from build123d import *

# Parameters (mm, degrees)
F1_DEPTH = 6.35
F2_R     = 0.762
F4_DEPTH = 6.3510001


with BuildPart() as f1:
    # F0 (on Top) → F1 (new body)
    with BuildSketch(Plane.XY):
        with BuildLine():
            Line((4.7625, 16.3680184094), (-4.7625, 16.3680184094))
            Line((-4.7625, 16.3680184094), (-4.7625, 11.2880184094))
            Line((-4.7625, 11.2880184094), (-1.27, 11.2880184094))
            Line((-1.27, 11.2880184094), (-1.27, 4.9380184094))
            ThreePointArc((-1.27, 4.9380184094), (-6.4291435291, 3.7546941592), (-10.16, 0))
            add(Edge.make_bspline(
                [(-8.7527767482, 0), (-8.8089559621, -0.2418498758), (-9.0471031461, -0.7278683078), (-10.0843877691, -0.5834050266), (-10.1370594903, -0.1969189085), (-10.16, 0)],
                knots=[0, 0, 0, 0, 0.3394019143, 0.707080255, 1, 1, 1, 1], degree=3))
            ThreePointArc((-8.7527767482, 0), (-5.3825469605, 2.5206872974), (-1.27, 3.4147067439))
            Line((-1.27, 3.4147067439), (-1.27, -12.192))
            Line((-1.27, -12.192), (-1.778, -12.192))
            Line((-1.778, -12.192), (-6.223, -3.556))
            Line((-6.223, -3.556), (-6.223, -1.27))
            Line((-6.223, -1.27), (-6.985, -1.27))
            Line((-6.985, -1.27), (-6.985, -3.556))
            Line((-6.985, -3.556), (-8.001, -3.556))
            Line((-8.001, -3.556), (-2.54, -13.716))
            Line((-2.54, -13.716), (2.54, -13.716))
            Line((2.54, -13.716), (8.001, -3.556))
            Line((8.001, -3.556), (6.985, -3.556))
            Line((6.985, -3.556), (6.985, -1.27))
            Line((6.985, -1.27), (6.223, -1.27))
            Line((6.223, -1.27), (6.223, -3.556))
            Line((6.223, -3.556), (1.778, -12.192))
            Line((1.778, -12.192), (1.27, -12.192))
            Line((1.27, -12.192), (1.27, 3.4147067439))
            ThreePointArc((1.27, 3.4147067439), (5.3825469605, 2.5206872974), (8.7527767482, 0))
            add(Edge.make_bspline(
                [(8.7527767482, 0), (8.8795025593, -0.2082938871), (9.0832410123, -0.668988318), (10.0510359017, -0.7151657897), (10.232657896, -0.2924908845), (10.16, 0)],
                knots=[0, 0, 0, 0, 0.3352638068, 0.68469439, 1, 1, 1, 1], degree=3))
            ThreePointArc((10.16, 0), (6.4291435291, 3.7546941592), (1.27, 4.9380184094))
            Line((1.27, 4.9380184094), (1.27, 11.2880184094))
            Line((1.27, 11.2880184094), (4.7625, 11.2880184094))
            Line((4.7625, 11.2880184094), (4.7625, 16.3680184094))
        make_face()
    extrude(amount=F1_DEPTH)

    # F2
    f2_edges = [f1.edges().sort_by_distance(p)[0] for p in [
        (-2.54, -13.716, 3.175),
        (2.54, -13.716, 3.175),
        (-4.7625, 16.368018, 3.175),
        (-4.7625, 11.288018, 3.175),
        (4.7625, 16.368018, 3.175),
        (4.7625, 11.288018, 3.175),
        (1.27, 3.414707, 3.175),
        (8.752777, 0, 3.175),
        (-8.752777, 0, 3.175),
        (-1.27, 3.414707, 3.175),
    ]]
    fillet(f2_edges, radius=F2_R)

    # F3 (on face) → F4 (cut, through all)
    with BuildSketch(Plane.XY.offset(6.35)):
        with BuildLine():
            Line((-3.048, 12.2405184094), (3.048, 12.2405184094))
            ThreePointArc((3.048, 12.2405184094), (3.5868153673, 12.4637030421), (3.81, 13.0025184094))
            Line((3.81, 13.0025184094), (3.81, 14.6535184094))
            ThreePointArc((3.81, 14.6535184094), (3.5868153673, 15.1923337767), (3.048, 15.4155184094))
            Line((3.048, 15.4155184094), (-3.048, 15.4155184094))
            ThreePointArc((-3.048, 15.4155184094), (-3.5868153673, 15.1923337767), (-3.81, 14.6535184094))
            Line((-3.81, 14.6535184094), (-3.81, 13.0025184094))
            ThreePointArc((-3.81, 13.0025184094), (-3.5868153673, 12.4637030421), (-3.048, 12.2405184094))
        make_face()
    extrude(amount=-F4_DEPTH, mode=Mode.SUBTRACT)


solid = f1.part
For this review, take the finished solid that the model builds, in its own axes (mm). A direction names the side the tool comes from. Round coordinates to 2 decimals unless told otherwise and drop trailing zeros. Loops run counter-clockwise (first coordinate to the right, second up) from the corner with the lowest first, then second, coordinate; pieces in that order, holes last. Notation, with made-up numbers: (25.25, -6) - (40.25, -6) arc R14 cw to (40.25, 12) - close; hole circle Ø1 at (0.5, 58). An arc over 180 degrees is marked (long way). Use one line per item in the form item = value.
Item 1: Consider section B-B on y = -5. Write out the cut boundary in (x, z).
Answers:
outline = (-7.22, 0) - (-5.48, 0) - (-5.48, 6.35) - (-7.22, 6.35) - close; (-1.27, 0) - (1.27, 0) - (1.27, 6.35) - (-1.27, 6.35) - close; (5.48, 0) - (7.22, 0) - (7.22, 6.35) - (5.48, 6.35) - close
Item 2: For line 1 (X direction, y = -3, z = 0.75) (3 decimals); line 2 (X direction, y = -11.5, z = 2.75); line 3 (Y direction, x = -4.5, z = 4.25), list the stretches that pass through material, from the lowest coordinate up.
Answers:
line_1 = -6.985 to -6.223, -1.27 to 1.27, 6.223 to 6.985
line_2 = -3.73 to -2.13, -1.27 to 1.27, 2.13 to 3.73
line_3 = -10.07 to -6.9, 2.87 to 4.56, 11.47 to 16.18
Item 3: Consider section D-D on y = 10. Write out the cut boundary in (x, z).
Answers:
outline = (-1.27, 0) - (1.27, 0) - (1.27, 6.35) - (-1.27, 6.35) - close
Item 4: Clearance check with flat-ended pins moving along their axes: P1, Ø0.8, axis at x = -3, z = 3, coming from the -Y side; P2, Ø1.1, axis at y = -2.5, z = 3.5, coming from the +X side (3 decimals); P3, Ø1.1, axis at y = 14.5, z = 1.5, coming from the -X side. State where each tip first meets the part, or that it passes through.
Answers:
P1 = -13.52
P2 = 6.985
P3 = -4.76
Item 5: Mouldability with a two-part tool opening along Y and no side actions: class faces 1 (the flat face through (5.342, -8.504, 3.131)), 2 (the flat face through (0, 0, 0)), 3 (the cylindrical face through (-5.72, 2.36, 3.13)), 4 (the flat face through (-1.27, -5, 3)) as +Y half, -Y half, draft (parallel to the pull), parting line (faces both ways), or undercut.
Answers:
face_1 = -Y half
face_2 = draft
face_3 = undercut
face_4 = undercut
Item 6: Consider section C-C on x = 3.5. Write out the cut boundary in (y, z), then the cut area to 3 significant figures.
Answers:
outline = (-11.93, 0) - (-8.85, 0) - (-8.85, 6.35) - (-11.93, 6.35) - close; (3.16, 0) - (4.8, 0) - (4.8, 6.35) - (3.16, 6.35) - close; (11.29, 0) - (12.39, 0) - (12.39, 6.35) - (11.29, 6.35) - close; (15.27, 0) - (16.37, 0) - (16.37, 6.35) - (15.27, 6.35) - close
area = 44.0 mm^2
Item 7: Consider section A-A on x = 0.5. Write out the cut boundary in (y, z).
Answers:
outline = (-13.72, 0) - (12.24, 0) - (12.24, 6.35) - (-13.72, 6.35) - close; (15.42, 0) - (16.37, 0) - (16.37, 6.35) - (15.42, 6.35) - close
Item 8: Tool access review of faces 5 (the flat face through (1.27, -5, 3)), 6 (the flat face through (4.762, 14, 3)), 7 (the flat face through (7.5, -3.556, 3.1)): name each direction out of +Z, -Z, +X, -X, +Y, -Y from which nothing blocks a thin tool from reaching the whole face with its end or side.
Answers:
face_5 = +Z, -Z
face_6 = +Z, -Z, +X, +Y
face_7 = +Z, -Z, +X
